Here's how the part is built. I have some questions about the finished solid (model axes, mm). A direction names the side the tool comes from. Round coordinates to 2 decimals unless told otherwise and drop trailing zeros. Write each loop counter-clockwise with the first axis right and the second up, starting at its lowest first coordinate (ties: lowest second). Pieces come first, ordered by that corner, then holes. Notation, with made-up numbers: M 77.5,-14.75 L 82.5,-14.75 A11 ccw 82.5,3.25 Z; hole C 29,-26.5 d3. An arc over 180 degrees is marked long. Use a Markdown table: item, result. Add a question column.
```python
from build123d import *

# Parameters (mm, degrees)
SKETCH1_R           = 3
BOSS_EXTRUDE1_DEPTH = 96.2
SKETCH2_W           = 629.4
SKETCH2_H           = 85
CUT_EXTRUDE1_DEPTH  = 93.2
LPATTERN1_COUNT     = 5
LPATTERN1_PITCH     = 88
CUT_EXTRUDE3_DEPTH  = 93.2
CUT_EXTRUDE4_DEPTH  = 3
CUT_EXTRUDE5_DEPTH  = 3
CUT_EXTRUDE6_DEPTH  = 3


with BuildPart() as part:
    # Sketch1 → Boss-Extrude1 (new body)
    with BuildSketch(Plane.XY):
        with BuildLine():
            Line((0, 0), (0, 206.5))
            ThreePointArc((0, 206.5), (15, 221.5), (0, 236.5))
            Line((0, 236.5), (0, 443))
            Line((0, 443), (-90.9, 443))
            ThreePointArc((-90.9, 443), (-105.9, 458), (-120.9, 443))
            Line((-120.9, 443), (-302.7, 443))
            ThreePointArc((-302.7, 443), (-317.7, 458), (-332.7, 443))
            Line((-332.7, 443), (-514.5, 443))
            ThreePointArc((-514.5, 443), (-529.5, 458), (-544.5, 443))
            Line((-544.5, 443), (-635.4, 443))
            Line((-635.4, 443), (-668.4, 415.309712171))
            Line((-668.4, 415.309712171), (-668.4, 236.5))
            ThreePointArc((-668.4, 236.5), (-683.4, 221.5), (-668.4, 206.5))
            Line((-668.4, 206.5), (-668.4, 27.690287829))
            Line((-668.4, 27.690287829), (-635.4, 0))
            Line((-635.4, 0), (-544.5, 0))
            ThreePointArc((-544.5, 0), (-529.5, -15), (-514.5, 0))
            Line((-514.5, 0), (-332.7, 0))
            ThreePointArc((-332.7, 0), (-317.7, -15), (-302.7, 0))
            Line((-302.7, 0), (-120.9, 0))
            ThreePointArc((-120.9, 0), (-105.9, -15), (-90.9, 0))
            Line((-90.9, 0), (0, 0))
        make_face()
        with Locations(Location((-529.5, 450.5, 0), (0, 0, 180))):
            Circle(SKETCH1_R, mode=Mode.SUBTRACT)
        with Locations(Location((-317.7, 450.5, 0), (0, 0, 180))):
            Circle(SKETCH1_R, mode=Mode.SUBTRACT)
        with Locations(Location((-105.9, 450.5, 0), (0, 0, 180))):
            Circle(SKETCH1_R, mode=Mode.SUBTRACT)
        with Locations(Location((7.5, 221.5, 0), (0, 0, 180))):
            Circle(SKETCH1_R, mode=Mode.SUBTRACT)
        with Locations(Location((-675.9, 221.5, 0), (0, 0, 180))):
            Circle(SKETCH1_R, mode=Mode.SUBTRACT)
        with Locations(Location((-529.5, -7.5, 0), (0, 0, 180))):
            Circle(SKETCH1_R, mode=Mode.SUBTRACT)
        with Locations(Location((-317.7, -7.5, 0), (0, 0, 180))):
            Circle(SKETCH1_R, mode=Mode.SUBTRACT)
        with Locations(Location((-105.9, -7.5, 0), (0, 0, 180))):
            Circle(SKETCH1_R, mode=Mode.SUBTRACT)
    extrude(amount=BOSS_EXTRUDE1_DEPTH)

    # Sketch2 → Cut-Extrude1 (cut)
    with BuildSketch(Plane.XY.offset(96.2)):
        with Locations((-317.7, 397.5)):
            Rectangle(SKETCH2_W, SKETCH2_H)
    cut_extrude1 = extrude(amount=-CUT_EXTRUDE1_DEPTH, mode=Mode.SUBTRACT)

    # LPattern1: Cut-Extrude1 ×5
    with Locations(*[(0, -i * LPATTERN1_PITCH, 0) for i in range(1, LPATTERN1_COUNT)]):
        add(cut_extrude1, mode=Mode.SUBTRACT)

    # Sketch5 → Cut-Extrude3 (cut)
    with BuildSketch(Plane.XY.offset(96.2)):
        Polygon((-665.4, 415.309712171), (-665.4, 27.690287829), (-635.4, 3), (-635.4, 440), align=None)
    extrude(amount=-CUT_EXTRUDE3_DEPTH, mode=Mode.SUBTRACT)

    # Sketch7 → Cut-Extrude4 (cut)
    with BuildSketch(Plane(origin=(0, 0, 0), x_dir=(0, 0, -1), z_dir=(1, 0, 0))):
        with BuildLine():
            Line((-69.2, 418), (-69.2, 246.5))
            ThreePointArc((-69.2, 246.5), (-71.2, 244.5), (-73.2, 246.5))
            Line((-73.2, 246.5), (-73.2, 418))
            ThreePointArc((-73.2, 418), (-71.2, 420), (-69.2, 418))
        make_face()
        with BuildLine():
            Line((-23, 418), (-23, 246.5))
            ThreePointArc((-23, 246.5), (-25, 244.5), (-27, 246.5))
            Line((-27, 246.5), (-27, 418))
            ThreePointArc((-27, 418), (-25, 420), (-23, 418))
        make_face()
        with BuildLine():
            Line((-69.2, 196.5), (-69.2, 25))
            ThreePointArc((-69.2, 25), (-71.2, 23), (-73.2, 25))
            Line((-73.2, 25), (-73.2, 196.5))
            ThreePointArc((-73.2, 196.5), (-71.2, 198.5), (-69.2, 196.5))
        make_face()
        with BuildLine():
            Line((-23, 196.5), (-23, 25))
            ThreePointArc((-23, 25), (-25, 23), (-27, 25))
            Line((-27, 25), (-27, 196.5))
            ThreePointArc((-27, 196.5), (-25, 198.5), (-23, 196.5))
        make_face()
    extrude(amount=-CUT_EXTRUDE4_DEPTH, mode=Mode.SUBTRACT)

    # Sketch8 → Cut-Extrude5 (cut)
    with BuildSketch(Plane.ZY.offset(635.4)):
        with BuildLine():
            Line((50.1, 415), (50.1, 28))
            ThreePointArc((50.1, 28), (48.1, 26), (46.1, 28))
            Line((46.1, 28), (46.1, 415))
            ThreePointArc((46.1, 415), (48.1, 417), (50.1, 415))
        make_face()
    extrude(amount=-CUT_EXTRUDE5_DEPTH, mode=Mode.SUBTRACT)

    # Sketch9 → Cut-Extrude6 (cut)
    with BuildSketch(Plane.ZY.offset(668.4)):
        with BuildLine():
            Line((50.1, 390.309712171), (50.1, 52.690287829))
            ThreePointArc((50.1, 52.690287829), (48.1, 50.690287829), (46.1, 52.690287829))
            Line((46.1, 52.690287829), (46.1, 390.309712171))
            ThreePointArc((46.1, 390.309712171), (48.1, 392.309712171), (50.1, 390.309712171))
        make_face()
    extrude(amount=-CUT_EXTRUDE6_DEPTH, mode=Mode.SUBTRACT)


solid = part.part
```
Item 1: Imagine slicing it at C-C on x = -418.5. List the corners of the cut face in (y, z) for me, plus the area to 3 significant figures.
Item 2: If we mould it in two halves opening along X, with no side actions, what happens to faces 1 (the face through (0, 102, 47)), 2 (the face through (-322, 267, 50)), 3 (the face through (-651.67, 429.35, 47.43)), 4 (the face through (-339, 225, 0))? For each: +X half, -X half, draft (parallel to the pull), parting line (faces both ways), or undercut.
Item 3: Imagine slicing it at A-A on y = 405. List the corners of the cut face in (x, z) for me, plus the area to 3 significant figures.
Item 4: On a 3-axis mill with a long thin cutter (end or side, diameter ignored), from which of +Z, -Z, +X, -X, +Y, -Y can I reach the whole of each face in a straight line? I mean faces 5 (the face through (-106, 458, 47)), 6 (the face through (-3, 309, 13)). Say none if no direction works.
Item 5: For pin 1 Ø4 at (x, z) = (-602, 68.5) entering from -Y; pin 2 Ø5 at (y, z) = (323, 44) entering from -X; pin 3 Ø2 at (x, z) = (-494.5, 77.5) entering from +Y, each with a flat end and sliding along its axis, tell me the tip position at first contact or that it passes through.
Item 6: I need wall thicknesses on probe 1 along Y at (x, z) = (-254.5, 43); probe 2 along X at (y, z) = (55.5, 55); probe 3 along X at (y, z) = (221.5, 76). Which ranges of each line are inside material? Lowest first, please. Write a range as from..to.
Item 7: Imagine slicing it at B-B on y = 339.5. List the corners of the cut face in (x, z) for me, plus the area to 3 significant figures.
Item 8: Imagine slicing it at D-D on z = 57. Count the separate pieces of the cut face and the enclosed holes in it, plus the area to 3 significant figures.
The answers:
| question | item | result |
|---|---|---|
| 1 | outline | M 0,0 L 443,0 L 443,96.2 L 440,96.2 L 440,3 L 355,3 L 355,96.2 L 352,96.2 L 352,3 L 267,3 L 267,96.2 L 264,96.2 L 264,3 L 179,3 L 179,96.2 L 176,96.2 L 176,3 L 91,3 L 91,96.2 L 88,96.2 L 88,3 L 3,3 L 3,96.2 L 0,96.2 Z |
| 1 | area | 3,010 mm² |
| 2 | face 1 | +X half |
| 2 | face 2 | undercut |
| 2 | face 3 | -X half |
| 2 | face 4 | draft |
| 3 | outline | M -668.4,0 L 0,0 L 0,23 L -3,23 L -3,3 L -632.4,3 L -632.4,46.1 L -635.4,46.1 L -635.4,3 L -665.4,3 L -665.4,96.2 L -668.4,96.2 Z; M -635.4,50.1 L -632.4,50.1 L -632.4,96.2 L -635.4,96.2 Z; M -3,27 L 0,27 L 0,69.2 L -3,69.2 Z; M -3,73.2 L 0,73.2 L 0,96.2 L -3,96.2 Z |
| 3 | area | 2,810 mm² |
| 4 | face 5 | +Z, -Z, +Y |
| 4 | face 6 | +Z |
| 5 | pin 1 | y = 0 |
| 5 | pin 2 | x = -668.4 |
| 5 | pin 3 | y = 443 |
| 6 | probe 1 | 0..3, 88..91, 176..179, 264..267, 352..355, 440..443 |
| 6 | probe 2 | -668.4..-665.4, -635.4..-632.4, -3..0 |
| 6 | probe 3 | -683.4..-678.9, -672.9..-665.4, -635.4..-632.4, -3..4.5, 10.5..15 |
| 7 | outline | M -668.4,0 L 0,0 L 0,23 L -3,23 L -3,3 L -632.4,3 L -632.4,46.1 L -635.4,46.1 L -635.4,3 L -665.4,3 L -665.4,46.1 L -668.4,46.1 Z; M -668.4,50.1 L -665.4,50.1 L -665.4,96.2 L -668.4,96.2 Z; M -635.4,50.1 L -632.4,50.1 L -632.4,96.2 L -635.4,96.2 Z; M -3,27 L 0,27 L 0,69.2 L -3,69.2 Z; M -3,73.2 L 0,73.2 L 0,96.2 L -3,96.2 Z |
| 7 | area | 2,800 mm² |
| 8 | separate pieces | 1 |
| 8 | enclosed holes | 14 |
| 8 | area | 17,900 mm² |
